Geometry check sheet. Reference: the model listing, model coordinates, mm. Face numbers are marked on the shaded views. A direction names the side the tool comes from. Round coordinates to 2 decimals unless told otherwise and drop trailing zeros. Write each loop counter-clockwise with the first axis right and the second up, starting at its lowest first coordinate (ties: lowest second). Pieces come first, ordered by that corner, then holes. Notation, with made-up numbers: (22, -13) - (54, -13) arc R28 ccw to (54, 9) - close; hole circle Ø3 at (18, 47.25). An arc over 180 degrees is marked (long way). Return JSON: item names as keys, results as strings. Group by question number.
from build123d import *

# Parameters (mm, degrees)
BOSS_EXTRUDE1_DEPTH = 6.35
SKETCH3_R           = 5.08
CUT_EXTRUDE3_DEPTH  = 6.35


with BuildPart() as part:
    # Sketch2 → Boss-Extrude1 (new body)
    with BuildSketch(Plane(origin=(0, 0, 0), x_dir=(1, 0, 0), z_dir=(0, 1, 0))):
        Polygon((-9.525, 16.497783942), (-9.525, 22.995384182), (-4.930502809, 18.400886991), (-3.24880012, 24.677086871), (0, 19.05), (3.24880012, 24.677086871), (4.930502809, 18.400886991), (9.525, 22.995384182), (9.525, 16.497783942), (15.152086871, 19.746584062), (13.470384182, 13.470384182), (19.746584062, 15.152086871), (16.497783942, 9.525), (22.995384182, 9.525), (18.400886991, 4.930502809), (24.677086871, 3.24880012), (19.05, 0), (24.677086871, -3.24880012), (18.400886991, -4.930502809), (22.995384182, -9.525), (16.497783942, -9.525), (19.746584062, -15.152086871), (13.470384182, -13.470384182), (15.152086871, -19.746584062), (9.525, -16.497783942), (9.525, -22.995384182), (4.930502809, -18.400886991), (3.24880012, -24.677086871), (0, -19.05), (-3.24880012, -24.677086871), (-4.930502809, -18.400886991), (-9.525, -22.995384182), (-9.525, -16.497783942), (-15.152086871, -19.746584062), (-13.470384182, -13.470384182), (-19.746584062, -15.152086871), (-16.497783942, -9.525), (-22.995384182, -9.525), (-18.400886991, -4.930502809), (-24.677086871, -3.24880012), (-19.05, 0), (-24.677086871, 3.24880012), (-18.400886991, 4.930502809), (-22.995384182, 9.525), (-16.497783942, 9.525), (-19.746584062, 15.152086871), (-13.470384182, 13.470384182), (-15.152086871, 19.746584062), align=None)
    extrude(amount=BOSS_EXTRUDE1_DEPTH)

    # Sketch3 → Cut-Extrude3 (cut)
    with BuildSketch(Plane(origin=(0, 6.35, 0), x_dir=(1, 0, 0), z_dir=(0, 1, 0))):
        with Locations(Location((0, 0, 0), (0, 0, 270))):
            Circle(SKETCH3_R)
    extrude(amount=-CUT_EXTRUDE3_DEPTH, mode=Mode.SUBTRACT)


solid = part.part
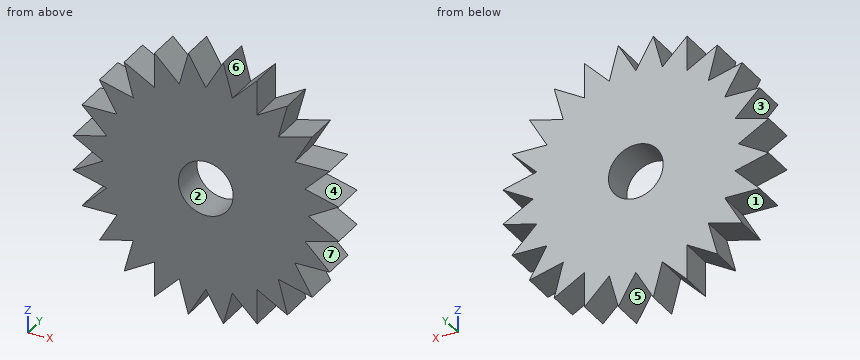
1. Tool access check on the marked faces 5, 6 and 7. Record the directions out of +Z, -Z, +X, -X, +Y, -Y that give a thin tool (end or side, any length) a straight path to the whole face; none if there is none.
2. Depth check by flat-ended pin: pin 1 Ø1.9 at (y, z) = (1.5, 20.5) entering from -X; pin 2 Ø3 at (y, z) = (1.5, 20) entering from +X; pin 3 Ø3 at (y, z) = (2, -1.5) entering from +X. Enter the tip coordinate at first touch or a pass-through.
3. Mould release check, pull along X, two halves, no side actions. Record for the marked faces 1, 2, 3 and 4: pulls with the +X half, pulls with the -X half, needs draft (parallel to the pull), parting line crosses it, or undercut.
4. Section check B-B (x = -2.5). Enter the section's corners in (y, z), and give its area (3 significant figures).
5. Material ranges on line 1 along X through (y, z) = (6.25, 17) (3 decimals); line 2 along Z through (x, y) = (22.5, 3.25) (3 decimals); line 3 along X through (y, z) = (6.25, -17.5) (3 decimals), recorded low to high.
6. Section check C-C (z = -20.5). Enter the section's corners in (x, y) (3 decimals).
7. Section check A-A (z = -2.5). Enter the section's corners in (x, y).
Result sheet:
{
 "1": {"face 5": "-Z, +Y, -Y", "face 6": "+Z, +Y, -Y", "face 7": "+X, +Y, -Y"},
 "2": {"pin 1": "stops at x = -15.15", "pin 2": "stops at x = 15.15", "pin 3": "stops at x = 24.25"},
 "3": {"face 1": "needs draft", "face 2": "undercut", "face 3": "pulls with the -X half", "face 4": "pulls with the +X half"},
 "4": {"outline": "(0, -23.38) - (6.35, -23.38) - (6.35, -4.42) - (0, -4.42) - close; (0, 4.42) - (6.35, 4.42) - (6.35, 23.38) - (0, 23.38) - close", "area": "241 mm²"},
 "5": {"line 1": "x = -14.416 to -10.395, -9.525 to 9.525, 10.395 to 14.416", "line 2": "z = -9.525 to -9.03, -3.832 to -1.992, 1.992 to 3.832, 9.03 to 9.525", "line 3": "x = -14.55 to -11.261, -9.525 to 9.525, 11.261 to 14.55"},
 "6": {"outline": "(-9.525, 0) - (-7.03, 0) - (-7.03, 6.35) - (-9.525, 6.35) - close; (-4.368, 0) - (-0.837, 0) - (-0.837, 6.35) - (-4.368, 6.35) - close; (0.837, 0) - (4.368, 0) - (4.368, 6.35) - (0.837, 6.35) - close; (7.03, 0) - (9.525, 0) - (9.525, 6.35) - (7.03, 6.35) - close"},
 "7": {"outline": "(-23.38, 0) - (-4.42, 0) - (-4.42, 6.35) - (-23.38, 6.35) - close; (4.42, 0) - (23.38, 0) - (23.38, 6.35) - (4.42, 6.35) - close"}
}
